```python
from build123d import *

# Parameters (mm, degrees)
F0_R     = 2.3114
F1_DEPTH = 50.8


with BuildPart() as f1:
    # F0 (on Top) → F1 (new body)
    with BuildSketch(Plane.XY):
        Polygon((3.031089, 1.75), (0, 3.5), (-3.031089, 1.75), (-3.031089, -1.75), (0, -3.5), (3.031089, -1.75), align=None)
        Circle(F0_R, mode=Mode.SUBTRACT)
    extrude(amount=F1_DEPTH)


with BuildPart() as f1_1:
    # F2: moved
    add(f1.part.moved(Location((0, 0, -25.4))))


solid = f1_1.part
```
Input: part model. Units: mm. Frame: model coordinates. Give positions to 0.01 mm unless a question says otherwise; leave off trailing zeros. Order: outer loops, then holes, each group sorted by start corner. A loop starts at its lowest first (then second) coordinate and runs counter-clockwise, first axis right, second up. Notation, with made-up numbers: (-4.5, -13) - (50.5, -13) arc R18 ccw to (50.5, -6) - close; hole circle Ø2 at (44, 54). An arc over 180 degrees is marked (long way). Use a Markdown table: item, result.
(1) Line query: line 1 (X direction, y = 1.5, z = 21); line 2 (Y direction, x = 0, z = 15); line 3 (Y direction, x = 0.75, z = 19). Output: solid intervals per line, ascending. Write a range as from..to.
Computed values:
| item | result |
|---|---|
| line 1 | x = -3.03..-1.76, 1.76..3.03 |
| line 2 | y = -3.5..-2.31, 2.31..3.5 |
| line 3 | y = -3.07..-2.19, 2.19..3.07 |
(2) Section query C-C (x = -0.5). Output: boundary loops of the cut face in (y, z), then the cut area to 3 significant figures.
Computed values:
| item | result |
|---|---|
| outline | (-3.21, -25.4) - (-2.26, -25.4) - (-2.26, 25.4) - (-3.21, 25.4) - close; (2.26, -25.4) - (3.21, -25.4) - (3.21, 25.4) - (2.26, 25.4) - close |
| area | 97.0 mm2 |
(3) Section query A-A (y = 0). Output: boundary loops of the cut face in (x, z).
Computed values:
| item | result |
|---|---|
| outline | (-3.03, -25.4) - (-2.31, -25.4) - (-2.31, 25.4) - (-3.03, 25.4) - close; (2.31, -25.4) - (3.03, -25.4) - (3.03, 25.4) - (2.31, 25.4) - close |
(4) Draft query along X for faces 1 (the cylindrical face through (-1.83, -1.41, -0.36)), 2 (the flat face through (3.031, 0, 0)), 3 (the flat face through (2, -2, -25.4)). Return one class per face: released by +X, released by -X, zero draft, split by the parting line, or undercut.
Computed values:
| item | result |
|---|---|
| face 1 | undercut |
| face 2 | released by +X |
| face 3 | zero draft |
(5) Pin query (flat end, axial travel): pin 1 (1.5 mm diameter, centred on x = 1.5, z = -18, fed in from -Y); pin 2 (1.5 mm diameter, centred on x = -2, z = -13.5, fed in from +Y). Return the tip coordinate at first contact, or that it passes through.
Computed values:
| item | result |
|---|---|
| pin 1 | stops at y = -3.07 |
| pin 2 | stops at y = 2.78 |
(6) Section query B-B (z = -15.5). Output: boundary loops of the cut face in (x, y), then the cut area to 3 significant figures.
Computed values:
| item | result |
|---|---|
| outline | (-3.03, -1.75) - (0, -3.5) - (3.03, -1.75) - (3.03, 1.75) - (0, 3.5) - (-3.03, 1.75) - close; hole circle Ø4.62 at (0, 0) |
| area | 15.0 mm2 |
